```python
from build123d import *

# Parameters (mm, degrees)
BOSS_EXTRUDE1_DEPTH  = 300
CHAMFER1_SIZE        = 0.5
SKETCH2_R            = 2.95
CUT_EXTRUDE1_DEPTH   = 5.6
LPATTERN1_COUNT      = 6
LPATTERN1_PITCH      = 25
LPATTERN2_COUNT      = 7
LPATTERN2_PITCH      = 25
SKETCH3_R            = 1.6
CUT_EXTRUDE2_DEPTH   = 9
LPATTERN3_COUNT      = 7
LPATTERN3_PITCH      = 25
LPATTERN3_COUNT_DIR2 = 6
LPATTERN3_PITCH_DIR2 = 25


with BuildPart() as part:
    # Sketch1 → Boss-Extrude1 (new body)
    with BuildSketch(Plane.XY):
        Polygon((6.05, 2.1), (3.95, 2.1), (3.95, 0.5), (6.05, 0.5), (6.05, -4), (-6.05, -4), (-6.05, 0.5), (-3.95, 0.5), (-3.95, 2.1), (-6.05, 2.1), (-6.05, 4), (6.05, 4), align=None)
    extrude(amount=BOSS_EXTRUDE1_DEPTH)

    # Chamfer1
    chamfer1_edges = [part.edges().sort_by_distance(p)[0] for p in [
        (6.05, -4, 150),
        (-6.05, -4, 150),
        (-6.05, 0.5, 150),
        (-6.05, 2.1, 150),
        (-6.05, 4, 150),
        (6.05, 4, 150),
        (6.05, 2.1, 150),
        (6.05, 0.5, 150),
    ]]
    chamfer(chamfer1_edges, length=CHAMFER1_SIZE)

    # Sketch2 → Cut-Extrude1 (cut)
    with BuildSketch(Plane(origin=(0, 4, 0), x_dir=(1, 0, 0), z_dir=(0, 1, 0))):
        with Locations((0, -137.5)):
            Circle(SKETCH2_R)
        with Locations((0, -162.5)):
            Circle(SKETCH2_R)
    cut_extrude1 = extrude(amount=-CUT_EXTRUDE1_DEPTH, mode=Mode.SUBTRACT)

    # LPattern1: Cut-Extrude1 ×6
    with Locations(*[(0, 0, i * LPATTERN1_PITCH) for i in range(1, LPATTERN1_COUNT)]):
        add(cut_extrude1, mode=Mode.SUBTRACT)

    # LPattern2: Cut-Extrude1 ×7
    with Locations(*[(0, 0, -i * LPATTERN2_PITCH) for i in range(1, LPATTERN2_COUNT)]):
        add(cut_extrude1, mode=Mode.SUBTRACT)

    # Sketch3 → Cut-Extrude2 (cut, through all)
    with BuildSketch(Plane(origin=(0, 4, 0), x_dir=(1, 0, 0), z_dir=(0, 1, 0))):
        with Locations((0, -162.5)):
            Circle(SKETCH3_R)
        with Locations((0, -137.5)):
            Circle(SKETCH3_R)
    cut_extrude2 = extrude(amount=-CUT_EXTRUDE2_DEPTH, mode=Mode.SUBTRACT)

    # LPattern3: Cut-Extrude2 7 × 6
    with Locations(*[Vector(0, 0, -1) * (i * LPATTERN3_PITCH) + Vector(0, 0, 1) * (j * LPATTERN3_PITCH_DIR2) for i in range(LPATTERN3_COUNT) for j in range(LPATTERN3_COUNT_DIR2) if (i, j) != (0, 0)]):
        add(cut_extrude2, mode=Mode.SUBTRACT)


solid = part.part
```
Read the model definition and answer for the solid it produces. Units are mm, in the model's axes. A direction names the side the tool comes from. Give positions to 0.01 mm unless a question says otherwise; leave off trailing zeros. Write each loop counter-clockwise with the first axis right and the second up, starting at its lowest first coordinate (ties: lowest second). Pieces come first, ordered by that corner, then holes. Notation, with made-up numbers: (83, 83) - (138, 83) arc R32 ccw to (138, 112) - close; hole circle Ø9 at (-22.75, -27). An arc over 180 degrees is marked (long way). Write item = value, one per line. Start each with the question number.
Item 1: A tool of negligible diameter and unlimited length cuts with its end or side. For faces 1 (the flat face through (0, -4, 148)), 2 (the cylindrical face through (-0.384, 1.239, 184.575)), from which of +Z, -Z, +X, -X, +Y, -Y can it reach the whole face along a straight path? Write none if from no direction.
Item 2: Each of these flat-tipped pins is pushed along its axis until it touches: P1, Ø3.5, axis at x = 0, z = 187.5, coming from the -Y side; P2, Ø5, axis at x = 0, z = 287.5, coming from the +Y side. Where does it stop, or does it pass through?
Item 3: Find the intervals of material crossed by probe 1 along X at (y, z) = (-2.1, 37.5); probe 2 along Y at (x, z) = (4, 47); probe 3 along X at (y, z) = (0.05, 237.5), in increasing order. Write a range as [from, to].
Item 4: Find section A-A (z = 147). Give the vertices of the cut face in (x, y), then the cut area to 3 significant figures.
Item 5: The mould has two halves that part along X. Classify faces 3 (the flat face through (0, 4, 148)), 4 (the cylindrical face through (-0.64, 1.24, 40.38)): +X half, -X half, draft (parallel to the pull), parting line (faces both ways), or undercut.
Response:
q1.face_1 = +Z, -Z, +X, -X, -Y
q1.face_2 = +Y
q2.P1 = -4
q2.P2 = -1.6
q3.probe_1 = [-6.05, -1.6], [1.6, 6.05]
q3.probe_2 = [-4, 0.5], [2.1, 4]
q3.probe_3 = [-6, -2.95], [2.95, 6]
q4.outline = (-6.05, -3.5) - (-5.55, -4) - (5.55, -4) - (6.05, -3.5) - (6.05, 0) - (5.55, 0.5) - (3.95, 0.5) - (3.95, 2.1) - (5.55, 2.1) - (6.05, 2.6) - (6.05, 3.5) - (5.55, 4) - (-5.55, 4) - (-6.05, 3.5) - (-6.05, 2.6) - (-5.55, 2.1) - (-3.95, 2.1) - (-3.95, 0.5) - (-5.55, 0.5) - (-6.05, 0) - close
q4.area = 89.1 mm²
q5.face_3 = draft
q5.face_4 = undercut
